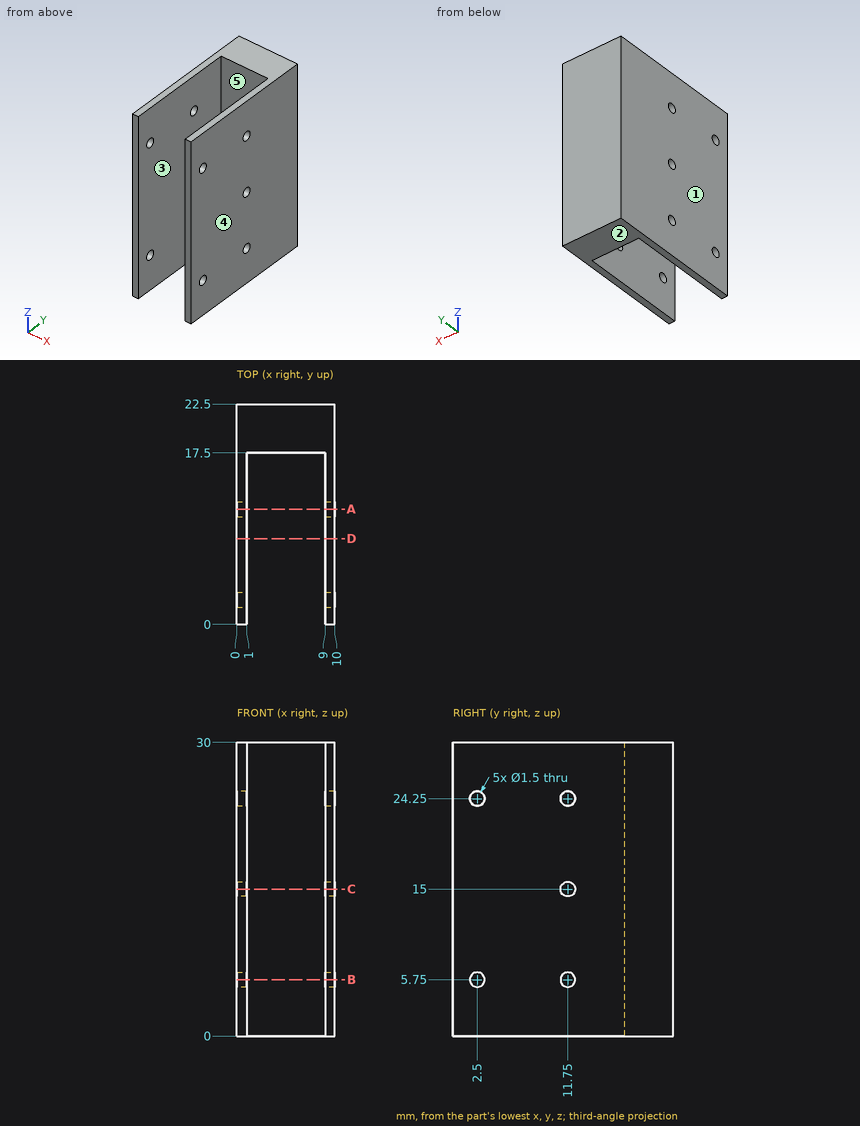
Here's the drawing with two shaded views (mm, measured from the low corner). I have some questions. A direction names the side the tool comes from. Round coordinates to 2 decimals unless told otherwise and drop trailing zeros. Loops run counter-clockwise (first coordinate to the right, second up) from the corner with the lowest first, then second, coordinate; pieces in that order, holes last.
1. Suppose I cut it at B-B, the plane z = 5.75. Please give me the cut outline in (x, y).
Answers:
outline: (0, 0) - (1, 0) - (1, 1.75) - (0, 1.75) - close; (0, 3.25) - (1, 3.25) - (1, 11) - (0, 11) - close; (0, 12.5) - (1, 12.5) - (1, 17.5) - (9, 17.5) - (9, 12.5) - (10, 12.5) - (10, 22.5) - (0, 22.5) - close; (9, 0) - (10, 0) - (10, 1.75) - (9, 1.75) - close; (9, 3.25) - (10, 3.25) - (10, 11) - (9, 11) - close
2. Suppose I cut it at D-D, the plane y = 8.75. Please give me the cut outline in (x, z).
Answers:
outline: (0, 0) - (1, 0) - (1, 30) - (0, 30) - close; (9, 0) - (10, 0) - (10, 30) - (9, 30) - close
3. If I drill on probe 1 along Y at (x, z) = (0.6, 24.25); probe 2 along X at (y, z) = (17, 11.25); probe 3 along Y at (x, z) = (9.85, 15), over which ranges is the centre line in solid material (lowest first)?
Answers:
probe 1: y = 0 to 1.75, 3.25 to 11, 12.5 to 22.5
probe 2: x = 0 to 1, 9 to 10
probe 3: y = 0 to 11, 12.5 to 22.5
4. Suppose I cut it at C-C, the plane z = 15. Please give me the cut outline in (x, y).
Answers:
outline: (0, 0) - (1, 0) - (1, 11) - (0, 11) - close; (0, 12.5) - (1, 12.5) - (1, 17.5) - (9, 17.5) - (9, 12.5) - (10, 12.5) - (10, 22.5) - (0, 22.5) - close; (9, 0) - (10, 0) - (10, 11) - (9, 11) - close
5. For the marked faces 4 and 5, which set-ups out of +Z, -Z, +X, -X, +Y, -Y let a thin tool reach every point of the face, with its end or its side?
Answers:
face 4: +Z, -Z, +X, +Y, -Y
face 5: +Z, -Z, -Y
6. Thinking about a two-plate mould opening in X: for the marked faces 1, 2 and 3, which applies, released by +X, released by -X, zero draft, split by the parting line, or undercut?
Answers:
face 1: released by -X
face 2: zero draft
face 3: undercut
7. Suppose I cut it at A-A, the plane y = 11.75. Give the number of separate pieces and of enclosed holes in the cut face, and give its area (3 significant figures).
Answers:
separate pieces: 8
enclosed holes: 0
area: 51.0 mm2
8. Will this pin go through, and if not, where does the flat tip stop? pin 1 (2 mm diameter, centred on x = 4.5, z = 19.5, fed in from -Y).
Answers:
pin 1: stops at y = 17.5
